Model file for the job. Use its own axes, mm. A direction names the side the tool comes from. Round coordinates to 2 decimals unless told otherwise and drop trailing zeros. Loops run counter-clockwise (first coordinate to the right, second up) from the corner with the lowest first, then second, coordinate; pieces in that order, holes last. Notation, with made-up numbers: (12.5, -6) - (31.5, -6) arc R20 cw to (31.5, 24) - close; hole circle Ø4 at (10, 77.25). An arc over 180 degrees is marked (long way). Answer as a JSON object with one key per item and string values.
from build123d import *

# Parameters (mm, degrees)
F0_R     = 1.75
F1_DEPTH = 3


# Not quite as in the source:
# - a feature names something its author has since deleted; it is built from what else it names


with BuildPart() as f1:
    # F0 (on Front) → F1 (new body)
    with BuildSketch(Plane.XZ):
        with BuildLine():
            Line((0, 16), (0, 0))
            Line((0, 0), (43.6382221521, 0))
            ThreePointArc((43.6382221521, 0), (43.870370626, 0.294923121), (44.1291400161, 0.5667888304))
            ThreePointArc((44.1291400161, 0.5667888304), (41.7991534918, 8.3522131948), (44.5474305371, 16))
            Line((44.5474305371, 16), (0, 16))
        make_face()
        with BuildLine():
            ThreePointArc((-9.8901239272, 4.9856294086), (-5.0141391128, 2.3557845503), (0, 0))
            Line((0, 0), (0, 16))
            ThreePointArc((0, 16), (-4.9775998147, 13.6626256025), (-9.8191881817, 11.0551668638))
            ThreePointArc((-9.8191881817, 11.0551668638), (-12.3290859965, 9.5638999576), (-14.7943813031, 8))
            ThreePointArc((-14.7943813031, 8), (-12.3639476772, 6.4575177277), (-9.8901239272, 4.9856294086))
        make_face()
        with BuildLine():
            Line((43.6382221521, 0), (0, 0))
            ThreePointArc((0, 0), (24.7921839108, -7.1853331257), (50.5976363139, -7.7853510181))
            ThreePointArc((50.5976363139, -7.7853510181), (49.8103733831, -6.7032232406), (49.4240926583, -5.4219853039))
            ThreePointArc((49.4240926583, -5.4219853039), (44.1587611024, -5.2426073702), (43.6382221521, 0))
        make_face()
        with BuildLine():
            ThreePointArc((80, 16), (40, 24.3484861009), (0, 16))
            Line((0, 16), (44.5474305371, 16))
            ThreePointArc((44.5474305371, 16), (54.7943813031, 21), (65.041332069, 16))
            Line((65.041332069, 16), (80, 16))
        make_face()
        with BuildLine():
            Line((-16, -0.0001621457), (-9.8901239272, 4.9856294086))
            ThreePointArc((-9.8901239272, 4.9856294086), (-12.3639476772, 6.4575177277), (-14.7943813031, 8))
            ThreePointArc((-14.7943813031, 8), (-12.3290859965, 9.5638999576), (-9.8191881817, 11.0551668638))
            Line((-9.8191881817, 11.0551668638), (-16, 16))
            Line((-16, 16), (-16, -0.0001621457))
        make_face()
        with BuildLine():
            ThreePointArc((44.5474305371, 16), (41.7991534918, 8.3522131948), (44.1291400161, 0.5667888304))
            ThreePointArc((44.1291400161, 0.5667888304), (47.2688331903, 1.6585032514), (50.1496109619, 0))
            Line((50.1496109619, 0), (58.9824606658, 0))
            ThreePointArc((58.9824606658, 0), (60.2984076368, 0.2226618407), (61.6143546079, 0))
            Line((61.6143546079, 0), (61.6856141113, 0))
            ThreePointArc((61.6856141113, 0), (63.1331562403, 3.9268000172), (67.289866632, 4.41351894))
            ThreePointArc((67.289866632, 4.41351894), (67.6676347628, 6.1891037132), (67.7943813031, 8))
            ThreePointArc((67.7943813031, 8), (67.0868659981, 12.2302269468), (65.041332069, 16))
            Line((65.041332069, 16), (44.5474305371, 16))
        make_face()
        with BuildLine():
            ThreePointArc((65.041332069, 16), (54.7943813031, 21), (44.5474305371, 16))
            Line((44.5474305371, 16), (65.041332069, 16))
        make_face()
        with BuildLine():
            Line((80, 0), (80, 16))
            Line((80, 16), (65.041332069, 16))
            ThreePointArc((65.041332069, 16), (67.0868659981, 12.2302269468), (67.7943813031, 8))
            ThreePointArc((67.7943813031, 8), (67.6676347628, 6.1891037132), (67.289866632, 4.41351894))
            ThreePointArc((67.289866632, 4.41351894), (68.9789922296, 2.9374861341), (69.6079694957, 0.7843011149))
            ThreePointArc((69.6079694957, 0.7843011149), (69.5885110127, 0.3902335683), (69.53032488, 0))
            Line((69.53032488, 0), (80, 0))
        make_face()
        with Locations((72.2943813031, 14)):
            Circle(F0_R, mode=Mode.SUBTRACT)
        with BuildLine():
            ThreePointArc((94.7943813031, 8), (87.5656775591, 12.3115824444), (80, 16))
            Line((80, 16), (80, 0))
            ThreePointArc((80, 0), (87.5656775591, 3.6884175556), (94.7943813031, 8))
        make_face()
        Polygon((-26, -11.0001621457), (-16, -0.0001621457), (-16, 16), (-26, 27), (-20.9564695358, 5.4488921514), align=None)
        with BuildLine():
            Line((58.9824606658, 0), (50.1496109619, 0))
            ThreePointArc((50.1496109619, 0), (50.6198306879, -0.8687025049), (50.862827722, -1.8261486257))
            ThreePointArc((50.862827722, -1.8261486257), (53.8241968939, -0.9475550969), (56.5284231629, -2.4404697788))
            ThreePointArc((56.5284231629, -2.4404697788), (57.4778318355, -0.941081445), (58.9824606658, 0))
        make_face()
        with BuildLine():
            ThreePointArc((63.935726955, -5.4416422713), (72.0834406348, -3.0620164808), (80, 0))
            Line((80, 0), (69.53032488, 0))
            ThreePointArc((69.53032488, 0), (67.5568042663, -2.7088411721), (64.215128062, -2.965364569))
            ThreePointArc((64.215128062, -2.965364569), (64.2775332757, -3.3692215709), (64.2984076368, -3.7773381593))
            ThreePointArc((64.2984076368, -3.7773381593), (64.2066858557, -4.6290196511), (63.935726955, -5.4416422713))
        make_face()
    extrude(amount=F1_DEPTH)


solid = f1.part
1) Slice it at A-A on z = 20. List the corners of the cut face in (x, y), then the cut area to 3 significant figures.
Values follow:
{"outline": "(-24.36, -3) - (-19.64, -3) - (-19.64, 0) - (-24.36, 0) - close; (10.83, -3) - (69.17, -3) - (69.17, 0) - (10.83, 0) - close", "area": "189 mm²"}
2) Tool access for faces 4 (the cylindrical face through (70.546, -1.479, 14.077)), 5 (the flat face through (-12.866, -1.479, 13.493)), 6 (the flat face through (-23.443, -1.479, -2.66)), 7 (the flat face through (-21.07, -1.48, -5.58)): list every direction of +Z, -Z, +X, -X, +Y, -Y with a clear straight run to the whole face (end or side of a thin tool).
Values follow:
{"face 4": "+Y, -Y", "face 5": "+Z, +Y, -Y", "face 6": "-X, +Y, -Y", "face 7": "-Z, +Y, -Y"}
3) Drop a flat-ended pin along its axis: P1, Ø1, axis at y = -1, z = -0.5, coming from the -X side. Give the stop position or say it passes through.
Values follow:
{"P1": "x = -22.93"}
4) Slice it at D-D on x = 25. List the corners of the cut face in (y, z).
Values follow:
{"outline": "(-3, -7.22) - (0, -7.22) - (0, 23.22) - (-3, 23.22) - close"}
5) Probe probe 1 along X at (y, z) = (-0.3, 15); probe 2 along Z at (x, y) = (0, -1.25); probe 3 along X at (y, z) = (-2.3, 12.5). List the from-to ranges inside material, lowest first.
Values follow:
{"probe 1": "-23.19 to -14.75, -2.22 to 70.86, 73.73 to 82.22", "probe 2": "0 to 16", "probe 3": "-22.61 to -11.63, -7.22 to 71.39, 73.2 to 87.22"}
6) Two-plate mould, pull along Z, no slides. Class faces 1 (the flat face through (34, -3, 8)), 2 (the flat face through (-12.988, -1.479, 2.458)), 3 (the flat face through (-23.514, -1.479, 16.375)): pulls with the +Z half, pulls with the -Z half, needs draft (parallel to the pull), parting line crosses it, or undercut.
Values follow:
{"face 1": "needs draft", "face 2": "pulls with the -Z half", "face 3": "undercut"}
7) Slice it at C-C on z = 14. List the corners of the cut face in (x, y), then the cut area to 3 significant figures.
Values follow:
{"outline": "(-22.96, -3) - (-13.5, -3) - (-13.5, 0) - (-22.96, 0) - close; (-4.3, -3) - (70.54, -3) - (70.54, 0) - (-4.3, 0) - close; (74.04, -3) - (84.3, -3) - (84.3, 0) - (74.04, 0) - close", "area": "284 mm²"}
8) Slice it at B-B on y = -0.5. List the corners of the cut face in (x, z).
Values follow:
{"outline": "(-26, -11) - (-16, 0) - (-9.89, 4.99) arc R100 ccw to (50.6, -7.79) arc R4 cw to (49.42, -5.42) arc R4 cw (long way) to (50.86, -1.83) arc R4 cw to (56.53, -2.44) arc R4 cw to (61.61, 0) - (61.69, 0) arc R4 cw (long way) to (64.22, -2.97) arc R4 cw to (63.94, -5.44) arc R100 ccw to (94.79, 8) arc R100 ccw to (-9.82, 11.06) - (-16, 16) - (-26, 27) - (-20.96, 5.45) - close; hole circle Ø3.5 at (72.29, 14)"}
